Check sheet for the modelled part. Datum: model origin and axes. Units: mm. A direction names the side the tool comes from. Coordinates: 2 decimals unless noted, no trailing zeros. Loops run counter-clockwise (first coordinate to the right, second up) from the corner with the lowest first, then second, coordinate; pieces in that order, holes last. Notation, with made-up numbers: (-12.5, -28) - (35.5, -28) arc R15 cw to (35.5, -6) - close; hole circle Ø6 at (-32.5, 3). An arc over 180 degrees is marked (long way). Use a Markdown table: item, result. Add a question column.
1) Sectioned sample at C-C, the plane z = 126. Enter the section's corners in (x, y) (3 decimals), then the cut area to 3 significant figures.
2) Tool access check on faces 1 (the cylindrical face through (-1.08, 4.88, -274.32)), 2 (the flat face through (0, 0, -280)), 3 (the cylindrical face through (-6, 0, 287)). Record the directions out of +Z, -Z, +X, -X, +Y, -Y that give a thin tool (end or side, any length) a straight path to the whole face; none if there is none.
3) Sectioned sample at D-D, the plane z = 275.5. Enter the section's corners in (x, y), then the cut area to 3 significant figures.
4) Go/stop test with flat-tipped pins: P1, Ø3, axis at x = -5, z = -35, coming from the +Y side; P2, Ø5, axis at y = 3, z = -214.5, coming from the +X side; P3, Ø5, axis at x = -5, z = 54, coming from the -Y side; P4, Ø1.5, axis at x = -1.5, y = -5, coming from the -Z side. Record where each tip stops, or that it passes through.
5) Thickness scan on line 1 (X direction, y = 1, z = 76.5); line 2 (Z direction, x = 5.75, y = 4); line 3 (Z direction, x = 5.75, y = -0.25). Record the ranges inside material, lowest first.
6) Sectioned sample at A-A, the plane y = 0. Enter the section's corners in (x, z) (3 decimals).
from build123d import *

# Parameters (mm, degrees)
F0_W   = 5
F0_H   = 15
F0_W_2 = 6
F0_H_2 = 22
F0_H_3 = 11
F3_R   = 0.2


# Not quite as in the source:
# - the program builds the solid bodies; features that only make, move or delete a surface that nothing else refers to are left out


with BuildPart() as f1:
    # F0 (on Front) → F1 (revolve)
    with BuildSketch(Plane.XZ):
        with Locations((2.5, 312.5)):
            Rectangle(F0_W, F0_H)
    revolve(axis=Axis((0, 0, -110.3163262457), (0, 0, -1)))



with BuildPart() as f1b:
    # F0 (on Front) → F1, piece 2 (revolve)
    with BuildSketch(Plane.XZ):
        with Locations((3, 280)):
            Rectangle(F0_W_2, F0_H_2)
        Polygon((0, 269), (0, 59.3673475087), (0, -269), (5, -269), (8.025, -269), (8.025, 269), (6, 269), align=None)
        with Locations((2.5, -274.5)):
            Rectangle(F0_W, F0_H_3)
    revolve(axis=Axis((0, 0, -110.3163262457), (0, 0, -1)))


with BuildPart() as f1_1:
    add(f1.part)

    add(f1b.part)  # F2 merges F1b
    # F0 (on Front) → F2 (revolve)
    with BuildSketch(Plane.XZ):
        Polygon((0, 305), (0, 291), (6, 291), (6, 305), (5, 305), align=None)
    revolve(axis=Axis((0, 0, 189.6836737543), (0, 0, 1)))

    # F3
    f3_edges = [f1_1.edges().sort_by_distance(p)[0] for p in [
        (-5, 0, -280),
    ]]
    fillet(f3_edges, radius=F3_R)


solid = f1_1.part
Solved:
| question | item | result |
|---|---|---|
| 1 | outline | circle Ø16.05 at (0, 0) |
| 1 | area | 202 mm2 |
| 2 | face 1 | -Z |
| 2 | face 2 | -Z, +X, -X, +Y, -Y |
| 2 | face 3 | +Z |
| 3 | outline | circle Ø12 at (0, 0) |
| 3 | area | 113 mm2 |
| 4 | P1 | stops at y = 7.22 |
| 4 | P2 | stops at x = 8.01 |
| 4 | P3 | stops at y = -7.63 |
| 4 | P4 | stops at z = -280 |
| 5 | line 1 | x = -7.96 to 7.96 |
| 5 | line 2 | z = -269 to 269 |
| 5 | line 3 | z = -269 to 305 |
| 6 | outline | (-8.025, -269) - (-5, -269) - (-5, -279.8) arc R0.2 ccw to (-4.8, -280) - (4.8, -280) arc R0.2 ccw to (5, -279.8) - (5, -269) - (8.025, -269) - (8.025, 269) - (6, 269) - (6, 305) - (5, 305) - (5, 320) - (-5, 320) - (-5, 305) - (-6, 305) - (-6, 269) - (-8.025, 269) - close |
